Could you check a few things on this model? Use its own coordinates, in mm. A direction names the side the tool comes from. Give positions to 0.01 mm unless a question says otherwise; leave off trailing zeros. Loops run counter-clockwise (first coordinate to the right, second up) from the corner with the lowest first, then second, coordinate; pieces in that order, holes last. Notation, with made-up numbers: M 79,7 L 121,7 A14 ccw 121,28 Z; hole C 61,-39.75 d7. An arc over 180 degrees is marked long. Use CSV: the item, a comma, the result in double quotes.
```python
from build123d import *

# Parameters (mm, degrees)
SKETCH1_R      = 1.59
EXTRUDE1_DEPTH = 3
SKETCH2_W      = 124
SKETCH2_H      = 30
EXTRUDE2_DEPTH = 3
SKETCH3_R      = 1.59
EXTRUDE3_DEPTH = 3


with BuildPart() as part:
    # Sketch1 → Extrude1 (new body)
    with BuildSketch(Plane(origin=(0, 0, 0), x_dir=(1, 0, 0), z_dir=(0, 1, 0))):
        Polygon((-6, 97.8583), (137.7752, 97.8583), (137.7752, -6), (137.7752, -9.96), (131.7752, -9.96), (0, -9.96), (-6, -9.96), (-6, -6), align=None)
        with Locations(Location((0, 91.8583, 0), (0, 0, 270))):
            Circle(SKETCH1_R, mode=Mode.SUBTRACT)
        with Locations(Location((131.7752, 91.8583, 0), (0, 0, 270))):
            Circle(SKETCH1_R, mode=Mode.SUBTRACT)
        with Locations(Location((131.7752, 0, 0), (0, 0, 270))):
            Circle(SKETCH1_R, mode=Mode.SUBTRACT)
        with Locations(Location((0, 0, 0), (0, 0, 270))):
            Circle(SKETCH1_R, mode=Mode.SUBTRACT)
    extrude(amount=-EXTRUDE1_DEPTH)

    # Sketch2 → Extrude2 (cut)
    with BuildSketch(Plane(origin=(0, 0, 0), x_dir=(1, 0, 0), z_dir=(0, 1, 0))):
        with Locations((65.8876, 82.8583)):
            Rectangle(SKETCH2_W, SKETCH2_H)
    extrude(amount=-EXTRUDE2_DEPTH, mode=Mode.SUBTRACT)

    # Sketch3 → Extrude3 (cut)
    with BuildSketch(Plane(origin=(0, 0, 0), x_dir=(1, 0, 0), z_dir=(0, 1, 0))):
        with Locations(Location((6.961270646, -7.468844026, 0), (0, 0, 270))):
            Circle(SKETCH3_R)
        with Locations(Location((6.970466443, 63.970156522, 0), (0, 0, 270))):
            Circle(SKETCH3_R)
        with Locations(Location((114.970465448, 63.956254506, 0), (0, 0, 270))):
            Circle(SKETCH3_R)
        with Locations(Location((114.96402933, 13.95625332, 0), (0, 0, 270))):
            Circle(SKETCH3_R)
        with Locations(Location((29, 13, 0), (0, 0, 270))):
            Circle(SKETCH3_R)
    extrude(amount=-EXTRUDE3_DEPTH, mode=Mode.SUBTRACT)


solid = part.part
```
1. I want a section at B-B, the plane x = 0. List the corners of the cut face in (y, z) for me.
Outcome:
outline,"M -3,-97.86 L 0,-97.86 L 0,-93.45 L -3,-93.45 Z; M -3,-90.27 L 0,-90.27 L 0,-1.59 L -3,-1.59 Z; M -3,1.59 L 0,1.59 L 0,9.96 L -3,9.96 Z"
2. Please list where these lines run through material, in increasing order: line 1 (X direction, y = -1.35, z = 0); line 2 (Z direction, x = 7, y = -0.85); line 3 (X direction, y = -1.15, z = -13).
Outcome:
line 1,"-6 to -1.59, 1.59 to 130.19, 133.37 to 137.78"
line 2,"-67.86 to -65.56, -62.38 to 5.88, 9.06 to 9.96"
line 3,"-6 to 27.41, 30.59 to 113.69, 116.23 to 137.78"
3. I'm going to push flat-ended pins straight in: pin 1 Ø4 at (x, z) = (0, -91.86) entering from +Y; pin 2 Ø1.5 at (x, y) = (43.5, -2) entering from -Z; pin 3 Ø1.9 at (x, z) = (0, 0) entering from -Y. Where does each tip first touch, or does it pass through?
Outcome:
pin 1,"y = 0"
pin 2,"z = -67.86"
pin 3,"through"
4. I want a section at C-C, the plane y = -0.6. Give the number of separate pieces and of enclosed holes in the cut face, then the cut area to 3 significant figures.
Outcome:
separate pieces,"1"
enclosed holes,"9"
area,"11,700 mm2"
5. I want a section at D-D, the plane z = -70.5. List the corners of the cut face in (x, y) for me, then the cut area to 3 significant figures.
Outcome:
outline,"M -6,-3 L 3.89,-3 L 3.89,0 L -6,0 Z; M 127.89,-3 L 137.78,-3 L 137.78,0 L 127.89,0 Z"
area,"59.3 mm2"
6. Which directions (+Z, -Z, +X, -X, +Y, -Y) give clear straight access to the entire face, cutting with the end or side of a thin tool? Please do faces 5 (the face through (127.888, -1, -83)), 6 (the face through (67, 0, -33)).
Outcome:
face 5,"-Z, +Y, -Y"
face 6,"+Z, -Z, +X, -X, +Y"
7. I want a section at A-A, the plane z = 0. List the corners of the cut face in (x, y) for me, then the cut area to 3 significant figures.
Outcome:
outline,"M -6,-3 L -1.59,-3 L -1.59,0 L -6,0 Z; M 1.59,-3 L 130.19,-3 L 130.19,0 L 1.59,0 Z; M 133.37,-3 L 137.78,-3 L 137.78,0 L 133.37,0 Z"
area,"412 mm2"
8. If we mould it in two halves opening along X, with no side actions, what happens to faces 1 (the face through (-6, -1, -45)), 2 (the face through (67, -3, -33)), 3 (the face through (65, -1, -67.858)), 4 (the face through (8.547, -1.479, -64.177))? For each: +X half, -X half, draft (parallel to the pull), parting line (faces both ways), or undercut.
Outcome:
face 1,"-X half"
face 2,"draft"
face 3,"undercut"
face 4,"undercut"
